For this review, take the finished solid that the model builds, in its own axes (mm). A direction names the side the tool comes from. Round coordinates to 2 decimals unless told otherwise and drop trailing zeros. Write each loop counter-clockwise with the first axis right and the second up, starting at its lowest first coordinate (ties: lowest second). Pieces come first, ordered by that corner, then holes.
Autodesk Inventor part; units mm, degrees
ref_plane "YZ Plane" through (0, 0, 0) normal (1, 0, 0) x (0, 1, 0)
ref_plane "XZ Plane" through (0, 0, 0) normal (0, 1, 0) x (-1, 0, 0)
ref_plane "XY Plane" through (0, 0, 0) normal (0, 0, 1) x (1, 0, 0)
sketch "Sketch1" plane through (0, 0, 0) normal (0, 1, 0) x (-1, 0, 0)
  circle A0 centre (0, 0) radius 25.0063
  circle A1 centre (0, 0) radius 21.082
  dimension "d0" = 50.0126
  dimension "d1" = 42.164
sketch "Sketch2" plane through (0, 0, 0) normal (0, 0, 1) x (1, 0, 0)
  line L0 (0, 0) -> (0, 36.068)
  line L1 (0, 36.068) -> (25.5039, 61.5719)
  line L2 (0, 36.068) -> (0, 32.2314) construction
  line L3 (-35.1083, 0) -> (35.606, 0) construction
  line L4 (25.0063, 0) -> (-25.0063, 0) construction
  dimension "d2" = 45
  dimension "d12" = 25.5039
  dimension "d13" = 36.068
  dimension "d14" = 61.5719
sweep "Sweep1" add profiles "Sketch1" path "Sketch2"
chamfer "Chamfer1" distance 3.175 angle 45 2 edges at (43.1861, 43.8898, 0) (25.0063, 0, 0)
equation "\"d12\" = 0.707107 * d13"
properties part number "Elbow 45degrees 1.25IN D" material "PVC-Piping"
(1) We need section B-B, the plane y = 19. Give the boundary of the cut face in (x, z), and give its area (3 significant figures).
Geometry check:
outline: circle Ø50.01 at (0, 0); hole circle Ø42.16 at (0, 0)
area: 568 mm2
(2) For line 1 along Z through (x, y) = (0, 30); line 2 along X through (y, z) = (30, -7), list the stretches that pass through material, from the lowest coordinate up.
Geometry check:
line 1: z = -25.01 to -21.08, 21.08 to 25.01
line 2: x = -24.01 to -19.89, 22.05 to 27.88
(3) Mouldability with a two-part tool opening along X and no side actions: class faces 1 (the face through (10.51, 76.29, -6.62)), 2 (the face through (4.8, 0.2, -21.5)), 3 (the face through (-20.11, 17.74, 6.33)), 4 (the face through (-0.813, 63.693, 6.332)) as pulls with the +X half, pulls with the -X half, needs draft (parallel to the pull), parting line crosses it, or undercut.
Geometry check:
face 1: pulls with the +X half
face 2: parting line crosses it
face 3: undercut
face 4: undercut
(4) We need section A-A, the plane z = 0. Give the boundary of the cut face in (x, y) (3 decimals), and give its area (3 significant figures).
Geometry check:
outline: (-25.006, 3.175) - (-21.831, 0) - (-21.082, 0) - (-21.082, 44.8) - (10.597, 76.479) - (10.067, 77.009) - (5.577, 77.009) - (-25.006, 46.426) - close; (21.082, 0) - (21.831, 0) - (25.006, 3.175) - (25.006, 25.71) - (40.941, 41.645) - (40.941, 46.135) - (40.411, 46.665) - (21.082, 27.336) - close
area: 546 mm2
(5) For faces 5 (the face through (-23.85, 20.3, 7.51)), 6 (the face through (20, 0, -8)), list the 3-axis set-ups (+Z, -Z, +X, -X, +Y, -Y) from which the entire face can be reached by the end or side of a thin tool; tool diameter is ignored.
Geometry check:
face 5: -Y
face 6: +Z, -Z, +X, -X, -Y
(6) For pin 1 Ø2 at (y, z) = (56.5, 16) entering from +X; pin 2 Ø1 at (x, z) = (4.5, -3) entering from -Y; pin 3 Ø2 at (x, z) = (3.5, -16.5) entering from -Y, all flat-tipped, find the tip position at first contact; note any pin that passes through.
Geometry check:
pin 1: stops at x = 3.05
pin 2: stops at y = 69.57
pin 3: stops at y = 55.97
